CAD build for the part. Positions are in the model's coordinates, mm. A direction names the side the tool comes from. Give positions to 0.01 mm unless a question says otherwise; leave off trailing zeros. Write each loop counter-clockwise with the first axis right and the second up, starting at its lowest first coordinate (ties: lowest second). Pieces come first, ordered by that corner, then holes. Notation, with made-up numbers: (-23, 46) - (0, 46) arc R20 ccw to (0, 63) - close; hole circle Ø6 at (15.25, 10). An arc over 180 degrees is marked (long way). Put each result on its own line as item: value. Start each with the question number.
1. Mould opens along X. For faces 1 (the flat face through (40.5, -1, 13)), 2 (the flat face through (-1, -32.5, 10)), 3 (the cylindrical face through (-34.521, 18.845, 13.944)), 4 (the flat face through (47.5, 0, 10)) say: +X half, -X half, draft (parallel to the pull), parting line (faces both ways), or undercut.
2. Wall check: line 1 (Y direction, x = -35, z = 14.5); line 2 (Y direction, x = 21, z = 9.25); line 3 (X direction, y = -24.5, z = 13.5). Give the ranges that are in metal, low to high.
3. Cut at C-C on x = -19.5. List the corners of the cut face in (y, z), and give its area (3 significant figures).
4. Tool access for faces 5 (the cylindrical face through (-39, 23, 11)), 6 (the cylindrical face through (-46.9, 31.93, 10.14)): list every direction of +Z, -Z, +X, -X, +Y, -Y with a clear straight run to the whole face (end or side of a thin tool).
5. Cut at D-D on y = -23. List the corners of the cut face in (x, z).
6. Cut at A-A on z = 15. Give the number of separate pieces and of enclosed holes in the cut face, and give its area (3 significant figures).
7. Cut at B-B on y = -1.5. List the corners of the cut face in (x, z), and give its area (3 significant figures).
8. Drop flat-ended pins along their axis: pin 1 (11 mm diameter, centred on x = -33, y = -18, fed in from +Z); pin 2 (2 mm diameter, centred on x = -35, y = -20, fed in from +Z); pin 3 (1.5 mm diameter, centred on x = 35, y = 20, fed in from +Z). Give the stop position or say it passes through.
Autodesk Inventor part; units mm, degrees
ref_plane "XY Plane" through (0, 0, 0) normal (0, 0, 1) x (1, 0, 0)
sketch "Sketch1" plane through (0, 0, 0) normal (0, 0, 1) x (1, 0, 0)
  line L0 (-47.5, -32.5) -> (47.5, -32.5)
  line L1 (47.5, -32.5) -> (47.5, 32.5)
  line L2 (47.5, 32.5) -> (-47.5, 32.5)
  line L3 (-47.5, 32.5) -> (-47.5, -32.5)
  point P0 (0, 0)
  point P1 (0, 32.5)
  point P2 (-47.5, 0)
  dimension "d0" = 65
  dimension "d1" = 95
extrude "Extrusion1" add sketch "Sketch1" along normal blind 20
sketch "Sketch4" plane through (0, 0, 20) normal (0, 0, 1) x (1, 0, 0)
  line L0 (-40.5, -25.7056) -> (40.5, -25.7056)
  line L1 (40.5, -25.7056) -> (40.5, 25.2944)
  line L2 (40.5, 25.2944) -> (-40.5, 25.2944)
  line L3 (-40.5, 25.2944) -> (-40.5, -25.7056)
  point P0 (0, 0)
  point P1 (0, 25.2944)
  point P2 (-40.5, -0.2056)
  dimension "d18" = 51
  dimension "d19" = 81
extrude "Extrusion3" cut sketch "Sketch4" against normal blind 15
sketch "Sketch5" plane through (0, 0, 5) normal (0, 0, 1) x (1, 0, 0)
  circle A0 centre (-35, 20) radius 5
  point P0 (0, 0)
  dimension "d22" = 10
  dimension "d23" = 35
  dimension "d24" = 20
extrude "Extrusion4" add sketch "Sketch5" along normal blind 13
sketch "Sketch6" plane through (-35, 20, 18) normal (0, 0, 1) x (1, 0, 0)
  circle A0 centre (0, 0) radius 5
  point P0 (35, -20)
hole "Hole2" at (-35, 20, 18) direction (0, 0, -1) diameter 2.5 depth 8 tip angle 118
mirror "Mirror3" about plane through (0, 0, 0) normal (1, 0, 0) of "Extrusion4", "Hole2"
mirror "Mirror4" about plane through (0, 0, 0) normal (0, 1, 0) of "Extrusion4", "Hole2", "Mirror3"
fillet "Fillet1" radius 2 4 edges at (47.5, 32.5, 10) (47.5, -32.5, 10) (-47.5, -32.5, 10) (-47.5, 32.5, 10)
properties part number "Case"
Report:
1. face 1: undercut
1. face 2: draft
1. face 3: undercut
1. face 4: +X half
2. line 1: y = -32.5 to -25.71, -25 to -21.25, -18.75 to -15, 15 to 18.75, 21.25 to 25, 25.29 to 32.5
2. line 2: y = -32.5 to -25.71, 25.29 to 32.5
2. line 3: x = -47.5 to -40.5, -37.18 to -32.82, 32.82 to 37.18, 40.5 to 47.5
3. outline: (-32.5, 0) - (32.5, 0) - (32.5, 20) - (25.29, 20) - (25.29, 5) - (-25.71, 5) - (-25.71, 20) - (-32.5, 20) - close
3. area: 535 mm²
4. face 5: +Z
4. face 6: +Z, -Z, -X, +Y
5. outline: (-47.5, 0) - (47.5, 0) - (47.5, 20) - (40.5, 20) - (40.5, 5) - (39, 5) - (39, 18) - (31, 18) - (31, 5) - (-31, 5) - (-31, 18) - (-39, 18) - (-39, 5) - (-40.5, 5) - (-40.5, 20) - (-47.5, 20) - close
6. separate pieces: 5
6. enclosed holes: 5
6. area: 2,340 mm²
7. outline: (-47.5, 0) - (47.5, 0) - (47.5, 20) - (40.5, 20) - (40.5, 5) - (-40.5, 5) - (-40.5, 20) - (-47.5, 20) - close
7. area: 685 mm²
8. pin 1: stops at z = 18
8. pin 2: stops at z = 9.85
8. pin 3: stops at z = 9.7
